Input: part model. Units: mm. Frame: model coordinates. A direction names the side the tool comes from. Round coordinates to 2 decimals unless told otherwise and drop trailing zeros. Loops run counter-clockwise (first coordinate to the right, second up) from the corner with the lowest first, then second, coordinate; pieces in that order, holes last. Notation, with made-up numbers: M 16.25,-37.5 L 26.25,-37.5 A13 cw 26.25,-32.5 Z; hole C 83,-11.5 d5. An arc over 180 degrees is marked long. Use one line per item in the form item = value. Start each with the question number.
Q1. First-contact query: P1, Ø5, axis at x = 94, y = 23.5, coming from the -Z side; P2, Ø9, axis at x = 132.5, y = 48.5, coming from the +Z side; P3, Ø1, axis at x = 104.5, y = 17.5, coming from the +Z side; P4, Ø8, axis at x = 80.327, z = 14.17, coming from the -Y side. Flat tips, straight axial feed; report the tip coordinate or a pass-through.
Q2. Section query C-C, the plane x = 17. Output: boundary loops of the cut face in (y, z), and give its area (3 significant figures).
Q3. Mould query, pull axis X, two halves, no side actions, for faces 1 (the flat face through (66, 1, 28)), 2 (the cylindrical face through (93.03, 1.48, 14.08)), 3 (the flat face through (143, 30, 14)). Classes: pulls with the +X half, pulls with the -X half, needs draft (parallel to the pull), parting line crosses it, or undercut.
Q4. Section query B-B, the plane x = 106.5. Output: boundary loops of the cut face in (y, z).
Q5. Section query A-A, the plane z = 23.5. Output: boundary loops of the cut face in (x, y), and give its area (3 significant figures).
Q6. Ray query, line 1 along Y through (x, z) = (10, 3.5); line 2 along X through (y, z) = (50, 3.3); line 3 along X through (y, z) = (32, 16.25). Return the intervals inside material, ascending.
Q7. Section query D-D, the plane y = 31. Output: boundary loops of the cut face in (x, z).
Q8. Access query for faces 4 (the flat face through (53, 1, 8.952)), 5 (the flat face through (132, 9, 6)), 6 (the cylindrical face through (134.155, 9.521, 2.958)). Directions: +Z, -Z, +X, -X, +Y, -Y. A direction counts if a zero-diameter tool reaches every point of the face in a straight line with its end or side. Return the directions, or none.
```python
from build123d import *

# Parameters (mm, degrees)
SKETCH_W        = 143
SKETCH_H        = 60
PAD_DEPTH       = 28
SKETCH002_W     = 137
SKETCH002_H     = 54
POCKET_DEPTH    = 25.001
SKETCH001_R     = 4
PAD001_DEPTH    = 6
SKETCH003_R     = 1.25
POCKET001_DEPTH = 28.001
SKETCH004_R     = 3.25
SKETCH004_R_2   = 3
SKETCH004_R_3   = 4.75
POCKET002_DEPTH = 5
SKETCH005_R     = 5
SKETCH005_R_2   = 6.5
POCKET003_DEPTH = 5


with BuildPart() as part:
    # Sketch → Pad (new body)
    with BuildSketch(Plane.XY):
        with Locations((71.5, 30)):
            Rectangle(SKETCH_W, SKETCH_H)
    extrude(amount=PAD_DEPTH)

    # Sketch002 → Pocket (cut, through all)
    with BuildSketch(Plane.XY.offset(3)):
        with Locations((71.5, 30)):
            Rectangle(SKETCH002_W, SKETCH002_H)
    extrude(amount=POCKET_DEPTH, mode=Mode.SUBTRACT)

    # Sketch001 → Pad001 (join)
    with BuildSketch(Plane.XY):
        with Locations((10, 50)):
            Circle(SKETCH001_R)
        with Locations((10, 10)):
            Circle(SKETCH001_R)
        with Locations((133, 50)):
            Circle(SKETCH001_R)
        with Locations((133, 10)):
            Circle(SKETCH001_R)
    extrude(amount=PAD001_DEPTH)

    # Sketch003 → Pocket001 (cut, through all)
    with BuildSketch(Plane.XY):
        with Locations((10, 10)):
            Circle(SKETCH003_R)
        with Locations((133, 10)):
            Circle(SKETCH003_R)
        with Locations((133, 50)):
            Circle(SKETCH003_R)
        with Locations((10, 50)):
            Circle(SKETCH003_R)
    extrude(amount=POCKET001_DEPTH, mode=Mode.SUBTRACT)

    # Sketch004 → Pocket002 (cut)
    with BuildSketch(Plane.XZ):
        with Locations((25, 12.67)):
            Circle(SKETCH004_R)
        with Locations((40.505, 13.9525)):
            Circle(SKETCH004_R_2)
        with Locations((65.495, 13.9525)):
            Circle(SKETCH004_R_2)
        with Locations((80.327, 14.17)):
            Circle(SKETCH004_R_3)
        with Locations((96.026, 13.9525)):
            Circle(SKETCH004_R_2)
        with Locations((121.016, 13.9525)):
            Circle(SKETCH004_R_2)
        with BuildLine():
            Line((46.549023, 8.9525), (59.450977, 8.9525))
            ThreePointArc((59.450977, 8.9525), (60.479437, 9.326829), (61.026669, 10.274663))
            Line((62.225692, 17.074663), (61.026669, 10.274663))
            ThreePointArc((62.225692, 17.074663), (61.875671, 18.38096), (60.65, 18.9525))
            Line((60.65, 18.9525), (45.35, 18.9525))
            ThreePointArc((45.35, 18.9525), (44.124329, 18.38096), (43.774308, 17.074663))
            Line((43.774308, 17.074663), (44.973331, 10.274663))
            ThreePointArc((44.973331, 10.274663), (45.520563, 9.326829), (46.549023, 8.9525))
        make_face()
        with BuildLine():
            Line((102.070023, 8.9525), (114.971977, 8.9525))
            ThreePointArc((114.971977, 8.9525), (116.000437, 9.326829), (116.547669, 10.274663))
            Line((117.746692, 17.074663), (116.547669, 10.274663))
            ThreePointArc((117.746692, 17.074663), (117.396671, 18.38096), (116.171, 18.9525))
            Line((116.171, 18.9525), (100.871, 18.9525))
            ThreePointArc((100.871, 18.9525), (99.645329, 18.38096), (99.295308, 17.074663))
            Line((99.295308, 17.074663), (100.494331, 10.274663))
            ThreePointArc((100.494331, 10.274663), (101.041563, 9.326829), (102.070023, 8.9525))
        make_face()
    extrude(amount=-POCKET002_DEPTH, mode=Mode.SUBTRACT)

    # Sketch005 → Pocket003 (cut)
    with BuildSketch(Plane.XZ):
        with Locations((25, 12.67)):
            Circle(SKETCH005_R)
        with Locations((80.327, 14.17)):
            Circle(SKETCH005_R_2)
    extrude(amount=-POCKET003_DEPTH, mode=Mode.SUBTRACT)


solid = part.part
```
Results found:
q1.P1 = 0
q1.P2 = 6
q1.P3 = 3
q1.P4 = 57
q2.outline = M 0,0 L 60,0 L 60,28 L 57,28 L 57,3 L 3,3 L 3,28 L 0,28 Z
q2.area = 330 mm²
q3.face_1 = needs draft
q3.face_2 = undercut
q3.face_3 = pulls with the +X half
q4.outline = M 0,0 L 60,0 L 60,28 L 57,28 L 57,3 L 3,3 L 3,8.95 L 0,8.95 Z; M 0,18.95 L 3,18.95 L 3,28 L 0,28 Z
q5.outline = M 0,0 L 143,0 L 143,60 L 0,60 Z; hole M 3,3 L 140,3 L 140,57 L 3,57 Z
q5.area = 1,180 mm²
q6.line_1 = 0 to 3, 6 to 8.75, 11.25 to 14, 46 to 48.75, 51.25 to 54, 57 to 60
q6.line_2 = 0 to 3, 6 to 8.75, 11.25 to 14, 129 to 131.75, 134.25 to 137, 140 to 143
q6.line_3 = 0 to 3, 140 to 143
q7.outline = M 0,0 L 143,0 L 143,28 L 140,28 L 140,3 L 3,3 L 3,28 L 0,28 Z
q8.face_4 = -Y
q8.face_5 = +Z
q8.face_6 = +Z, -Z
